```python
from build123d import *


with BuildPart() as part:
    # Sketch2 → Revolve1 (revolve)
    with BuildSketch(Plane(origin=(0, 0, 0), x_dir=(0, 0, -1), z_dir=(1, 0, 0))):
        with BuildLine():
            Line((-14.795, 9.374), (-14.795, 10.3791))
            ThreePointArc((-14.795, 10.3791), (-14.736421356, 10.520521356), (-14.595, 10.5791))
            Line((-14.595, 10.5791), (2.505, 10.5791))
            ThreePointArc((2.505, 10.5791), (2.646421356, 10.520521356), (2.705, 10.3791))
            Line((2.705, 10.3791), (2.705, 0))
            Line((2.705, 0), (0, 0))
            Line((0, 0), (0, 7.874))
            Line((0, 7.874), (-13.295, 7.874))
            Line((-13.295, 7.874), (-14.795, 9.374))
        make_face()
    revolve(axis=Axis((0, 0, -2.705), (0, 0, 1)))


solid = part.part
```
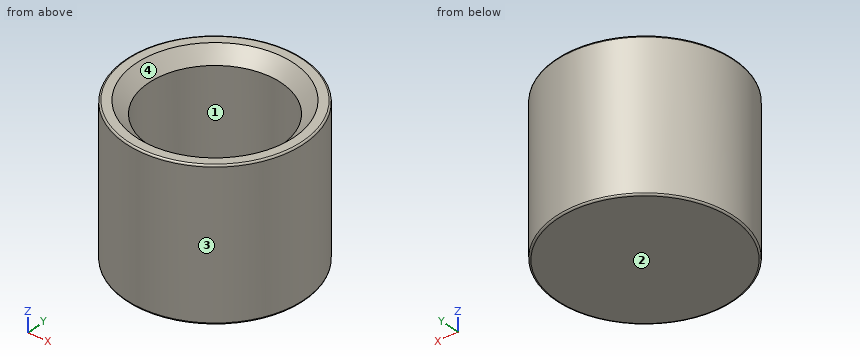
The model under review builds one solid part; all positions refer to its coordinate system, in mm. Face numbers are marked on the shaded views. Round coordinates to 2 decimals unless told otherwise and drop trailing zeros. Loops run counter-clockwise (first coordinate to the right, second up) from the corner with the lowest first, then second, coordinate; pieces in that order, holes last.
Item 1: Take a section at B-B (z = 2.5). Write out the cut boundary in (x, y).
Determined:
outline: circle Ø21.16 at (0, 0); hole circle Ø15.75 at (0, 0)
Item 2: Take a section at A-A (y = 0). Write out the cut boundary in (x, z) (3 decimals).
Determined:
outline: (-10.579, -2.505) arc R0.2 ccw to (-10.379, -2.705) - (10.379, -2.705) arc R0.2 ccw to (10.579, -2.505) - (10.579, 14.595) arc R0.2 ccw to (10.379, 14.795) - (9.374, 14.795) - (7.874, 13.295) - (7.874, 0) - (-7.874, 0) - (-7.874, 13.295) - (-9.374, 14.795) - (-10.379, 14.795) arc R0.2 ccw to (-10.579, 14.595) - close
Item 3: For line 1 (Y direction, x = 0, z = 4.75); line 2 (Z direction, x = -1, y = -3.5) (3 decimals), list the stretches that pass through material, from the lowest coordinate up.
Determined:
line 1: y = -10.58 to -7.87, 7.87 to 10.58
line 2: z = -2.705 to 0
Item 4: Mouldability with a two-part tool opening along Y and no side actions: class the marked faces 1, 2, 3 and 4 as released by +Y, released by -Y, zero draft, split by the parting line, or undercut.
Determined:
face 1: undercut
face 2: zero draft
face 3: split by the parting line
face 4: undercut
Item 5: Clearance check with flat-ended pins moving along their axes: pin 1 Ø5 at (x, y) = (1, 5) entering from +Z; pin 2 Ø5 at (y, z) = (5.5, 10.5) entering from -X; pin 3 Ø1 at (y, z) = (5, 7) entering from +X. State where each tip first meets the part, or that it passes through.
Determined:
pin 1: stops at z = 0
pin 2: stops at x = -10.14
pin 3: stops at x = 9.57
